Autodesk Inventor part; units mm, degrees
ref_plane "YZ Plane" through (0, 0, 0) normal (1, 0, 0) x (0, 1, 0)
ref_plane "XZ Plane" through (0, 0, 0) normal (0, 1, 0) x (-1, 0, 0)
ref_plane "XY Plane" through (0, 0, 0) normal (0, 0, 1) x (1, 0, 0)
sketch "Sketch1" plane through (0, 0, 0) normal (1, 0, 0) x (0, 1, 0)
  circle A0 centre (17.9578, -17.9578) radius 3.81
  circle A1 centre (35.9156, 0) radius 3.175
  circle A2 centre (0, -35.9156) radius 3.175
  circle A3 centre (35.9156, -35.9156) radius 3.175
  circle A4 centre (0, 0) radius 3.175
  line L0 (17.9578, -17.9578) -> (23.346, -23.346)
  line L1 (23.346, -23.346) -> (12.5696, -23.346)
  line L2 (17.9578, -28.7341) -> (37.7144, -48.4907)
  line L3 (37.7144, -48.4907) -> (48.4907, -37.7144)
  line L4 (48.4907, -37.7144) -> (28.7341, -17.9578)
  line L5 (17.9578, -28.7341) -> (-1.7988, -48.4907)
  line L6 (-1.7988, -48.4907) -> (-12.5751, -37.7144)
  line L7 (-12.5751, -37.7144) -> (7.1815, -17.9578)
  line L8 (7.1815, -17.9578) -> (-12.5751, 1.7988)
  line L9 (-12.5751, 1.7988) -> (-1.7988, 12.5751)
  line L10 (-1.7988, 12.5751) -> (17.9578, -7.1815)
  line L11 (17.9578, -7.1815) -> (37.7144, 12.5751)
  line L12 (37.7144, 12.5751) -> (48.4907, 1.7988)
  line L13 (48.4907, 1.7988) -> (28.7341, -17.9578)
  line L14 (35.9156, 0) -> (33.6705, -2.2451)
  line L15 (0, 0) -> (2.2451, -2.2451)
  line L16 (15.2637, -15.2637) -> (17.9578, -17.9578)
  line L17 (22.6724, -13.2432) -> (20.6519, -15.2637)
  line L18 (15.2637, -20.6519) -> (12.5696, -23.346)
  line L19 (2.2451, -33.6705) -> (0, -35.9156)
  line L20 (35.9156, 0) -> (35.9156, -3.175)
  line L21 (35.9156, -32.7406) -> (35.9156, -35.9156)
  line L22 (35.9156, -35.9156) -> (32.7406, -35.9156)
  line L23 (3.175, -35.9156) -> (0, -35.9156)
  line L24 (0, -35.9156) -> (0, -32.7406)
  line L25 (0, -3.175) -> (0, 0)
  line L26 (0, 0) -> (3.175, 0)
  line L27 (32.7406, 0) -> (35.9156, 0)
  point P0 (20.6519, -20.6519)
  dimension "d0" = 35.9156
  dimension "d1" = 35.9156
  dimension "d2" = 7.62
  dimension "d3" = 6.35
  dimension "d4" = 6.35
  dimension "d5" = 6.35
  dimension "d6" = 6.35
  dimension "d7" = 7.62
  dimension "d8" = 35.56
  dimension "d9" = 15.24
  dimension "d10" = 35.56
  dimension "d11" = 15.24
  dimension "d12" = 35.56
extrude "Extrusion1" add sketch "Sketch1" along normal blind 6.35 contours L0 L1 L18 A0 | L5 L6 L7 L8 L9 L10 L11 L12 L13 L4 L3 L2
fillet "Fillet1" radius 6.35 12 edges at (3.175, 28.7341, -17.9578) (3.175, 48.4907, -37.7144) (3.175, 37.7144, -48.4907) (3.175, -1.7988, -48.4907) (3.175, -1.7988, 12.5751) (3.175, 37.7144, 12.5751) (3.175, 48.4907, 1.7988) (3.175, 17.9578, -28.7341) (3.175, -12.5751, -37.7144) (3.175, -12.5751, 1.7988) (3.175, 7.1815, -17.9578) (3.175, 17.9578, -7.1815)
properties part number "Gearbox"
Work out the finished part from the listing and answer in its coordinate system (mm). A direction names the side the tool comes from. Round coordinates to 2 decimals unless told otherwise and drop trailing zeros. Loops run counter-clockwise (first coordinate to the right, second up) from the corner with the lowest first, then second, coordinate; pieces in that order, holes last. Notation, with made-up numbers: (63, 46) -> (81, 46) arc R24 ccw to (81, 75) -> close; hole circle Ø3 at (56, 13). An arc over 180 degrees is marked (long way). Use one line per item in the form item = value.
(1) Find section A-A on y = 0. Give the vertices of the cut face in (x, z) (3 decimals).
Answer list:
outline = (0, -45.6) -> (6.35, -45.6) -> (6.35, -39.091) -> (0, -39.091) -> close; (0, -32.741) -> (6.35, -32.741) -> (6.35, -25.139) -> (0, -25.139) -> close; (0, -10.776) -> (6.35, -10.776) -> (6.35, -3.175) -> (0, -3.175) -> close; (0, 3.175) -> (6.35, 3.175) -> (6.35, 9.685) -> (0, 9.685) -> close
(2) Find section D-D on x = 4. Give the number of separate pieces and of enclosed holes in the cut face, then the cut area to 3 significant figures.
Answer list:
separate_pieces = 1
enclosed_holes = 5
area = 1,730 mm2
(3) Flat-ended cylindrical pins translate along their axes: P1, Ø2, axis at x = 5.5, y = -4.5, coming from the +Z side; P2, Ø1.5, axis at x = 5, y = 25, coming from the +Z side; P3, Ø3, axis at x = 5, y = 6.5, coming from the -Z side. Find the tip coordinate at first contact, or state that the pin passes through.
Answer list:
P1 = 9.71
P2 = 0.61
P3 = -41.69
(4) A tool of negligible diameter and unlimited length cuts with its end or side. For faces 1 (the flat face through (3.131, 27.761, -38.537)), 2 (the cylindrical face through (3.22, 45.86, 1.73)), 3 (the flat face through (3.131, -2.621, -8.155)), 4 (the flat face through (3.131, 43.09, -43.115)), 5 (the flat face through (3.131, 8.004, 2.772)), from which of +Z, -Z, +X, -X, +Y, -Y can it reach the whole face along a straight path? Write none if from no direction.
Answer list:
face_1 = -Z, +X, -X
face_2 = +X, -X, +Y
face_3 = +X, -X, -Y
face_4 = -Z, +X, -X, +Y
face_5 = +Z, +X, -X
(5) Find section B-B on z = -16.5. Give the vertices of the cut face in (x, y), then the cut area to 3 significant figures.
Answer list:
outline = (0, 4.38) -> (6.35, 4.38) -> (6.35, 14.44) -> (0, 14.44) -> close; (0, 21.48) -> (6.35, 21.48) -> (6.35, 31.53) -> (0, 31.53) -> close
area = 128 mm2
(6) Find section C-C on y = 40. Give the vertices of the cut face in (x, z), then the cut area to 3 significant figures.
Answer list:
outline = (0, -45.43) -> (6.35, -45.43) -> (6.35, -29.22) -> (0, -29.22) -> close; (0, -6.69) -> (6.35, -6.69) -> (6.35, 9.52) -> (0, 9.52) -> close
area = 206 mm2
(7) For a pull along Z with two mould halves and no side action, classify faces 6 (the cylindrical face through (3.219, 18.028, -31.365)), 7 (the cylindrical face through (3.13, 14.15, -18.13)), 8 (the flat face through (3.131, -7.2, 7.174)) as released by +Z, released by -Z, zero draft, split by the parting line, or undercut.
Answer list:
face_6 = released by -Z
face_7 = undercut
face_8 = released by +Z
(8) Straight lines are drawn through the part: line 1 (Z direction, x = 5.75, y = 1); line 2 (Y direction, x = 5.25, z = 0) (3 decimals); line 3 (Y direction, x = 5.25, z = -34.5). For each, find the intervals that lie inside material, in ascending order.
Answer list:
line_1 = -45.21 to -38.93, -32.9 to -24.14, -11.78 to -3.01, 3.01 to 9.29
line_2 = -9.685 to -3.175, 3.175 to 10.776, 25.139 to 32.741, 39.091 to 45.6
line_3 = -9.07 to -2.84, 2.84 to 12.19, 23.72 to 33.07, 38.76 to 44.99
